```python
from build123d import *

# Parameters (mm, degrees)
LEAF_START           = 96
LEAF_DEPTH           = 28
SKETCH_2_R           = 3.3
MOUNTING_HOLES_DEPTH = 4


with BuildPart() as part:
    # 草图1 → Leaf (new body)
    with BuildSketch(Plane(origin=(0, 0, 0), x_dir=(0, 0, -1), z_dir=(1, 0, 0)).offset(LEAF_START)):
        Polygon((0.98338218, 40.181547479), (-23.01661782, 170.181547479), (-24.98338218, 169.818452521), (-0.98338218, 39.818452521), align=None)
    extrude(amount=LEAF_DEPTH)

    # 草图2 → Mounting Holes (cut, symmetric)
    with BuildSketch(Plane(origin=(0, 1.136832012, -6.157840067), x_dir=(1, 0, 0), z_dir=(0, -0.18154747945610336, 0.9833821803872266))):
        with Locations(Location((102, 52.335287215, 0), (0, 0, 270))):
            Circle(SKETCH_2_R)
        with Locations(Location((118, 52.335287215, 0), (0, 0, 270))):
            Circle(SKETCH_2_R)
        with Locations(Location((102, 158.532110173, 0), (0, 0, 270))):
            Circle(SKETCH_2_R)
        with Locations(Location((118, 158.532110173, 0), (0, 0, 270))):
            Circle(SKETCH_2_R)
    extrude(amount=MOUNTING_HOLES_DEPTH, both=True, mode=Mode.SUBTRACT)


solid = part.part
```
Geometry check sheet. Reference: the model listing, model coordinates, mm. Round coordinates to 2 decimals unless told otherwise and drop trailing zeros. Loops run counter-clockwise (first coordinate to the right, second up) from the corner with the lowest first, then second, coordinate; pieces in that order, holes last. Notation, with made-up numbers: (-38, 20.25) - (10, 20.25) arc R28 ccw to (10, 51.25) - close; hole circle Ø5 at (75.25, 65.5). An arc over 180 degrees is marked (long way). Write each question's results on one line, items separated by ' | '. Start each with the question number.
Q1. Cross-section at A-A on x = 116. Enter the section's corners in (y, z).
Q2. Thickness scan on line 1 (Z direction, x = 104.5, y = 61.5); line 2 (Z direction, x = 109.5, y = 59). Record the ranges inside material, lowest first. Write a range as [from, to].
Q3. Cross-section at B-B on x = 108.25. Enter the section's corners in (y, z).
Q4. Gauge pin test, flat ends, axial feed: P1, Ø4, axis at x = 118, y = 119, coming from the -Z side; P2, Ø10, axis at x = 114, y = 83, coming from the +Z side. Record the tip position at first contact, or that the pin passes through.
Q5. Cross-section at C-C on y = 138. Enter the section's corners in (x, z).
Q6. Release check for a two-part mould opening along X. For faces 1 (the flat face through (96, 105, 12)), 2 (the flat face through (124, 105, 12)), 3 (the flat face through (109.8, 105.73, 13.15)), 4 (the cylindrical face through (102.99, 154.12, 21.08)) record: +X half, -X half, draft (parallel to the pull), parting line (faces both ways), or undercut.
Answers below:
1) outline: (39.82, 0.98) - (40.18, -0.98) - (50.38, 0.9) - (50.02, 2.87) - close; (55.18, 3.82) - (55.55, 1.85) - (154.82, 20.18) - (154.45, 22.15) - close; (159.62, 23.1) - (159.98, 21.13) - (170.18, 23.02) - (169.82, 24.98) - close
2) line 1: z = [2.95, 4.99] | line 2: z = [2.49, 4.52]
3) outline: (39.82, 0.98) - (40.18, -0.98) - (170.18, 23.02) - (169.82, 24.98) - close
4) P1: stops at z = 13.2 | P2: stops at z = 9.88
5) outline: (96, 17.08) - (124, 17.08) - (124, 19.11) - (96, 19.11) - close
6) face 1: -X half | face 2: +X half | face 3: draft | face 4: undercut
